```python
from build123d import *

# Parameters (mm, degrees)
SKETCH1_W           = 41
SKETCH1_H           = 19.4
BOSS_EXTRUDE1_DEPTH = 20.3
SKETCH2_W           = 54.7
SKETCH2_H           = 20.3
BOSS_EXTRUDE2_DEPTH = 2.6
SKETCH3_W           = 41
SKETCH3_H           = 20.3
BOSS_EXTRUDE3_DEPTH = 6.6
SKETCH4_R           = 2.2
CUT_EXTRUDE1_DEPTH  = 57.442116367
SKETCH5_R           = 5
BOSS_EXTRUDE4_DEPTH = 0.7
SKETCH6_R           = 2.97
BOSS_EXTRUDE5_DEPTH = 4.3


with BuildPart() as part:
    # Sketch1 → Boss-Extrude1 (new body)
    with BuildSketch(Plane.XY):
        with Locations((20.5, -9.7)):
            Rectangle(SKETCH1_W, SKETCH1_H)
    extrude(amount=BOSS_EXTRUDE1_DEPTH)

    # Sketch2 → Boss-Extrude2 (add)
    with BuildSketch(Plane(origin=(0, 0, 0), x_dir=(1, 0, 0), z_dir=(0, 1, 0))):
        with Locations((20.5, -10.15)):
            Rectangle(SKETCH2_W, SKETCH2_H)
    extrude(amount=BOSS_EXTRUDE2_DEPTH)

    # Sketch3 → Boss-Extrude3 (add)
    with BuildSketch(Plane(origin=(0, 2.6, 0), x_dir=(1, 0, 0), z_dir=(0, 1, 0))):
        with Locations((20.5, -10.15)):
            Rectangle(SKETCH3_W, SKETCH3_H)
    extrude(amount=BOSS_EXTRUDE3_DEPTH)

    # Sketch4 → Cut-Extrude1 (cut, through all)
    with BuildSketch(Plane(origin=(0, 2.6, 0), x_dir=(1, 0, 0), z_dir=(0, 1, 0))):
        with Locations(Location((-4.4, -15.15, 0), (0, 0, 270))):
            Circle(SKETCH4_R)
        with Locations(Location((-4.4, -5.15, 0), (0, 0, 270))):
            Circle(SKETCH4_R)
        with Locations(Location((45.4, -15.15, 0), (0, 0, 270))):
            Circle(SKETCH4_R)
        with Locations(Location((45.4, -5.15, 0), (0, 0, 270))):
            Circle(SKETCH4_R)
    extrude(amount=-CUT_EXTRUDE1_DEPTH, mode=Mode.SUBTRACT)

    # Sketch5 → Boss-Extrude4 (add)
    with BuildSketch(Plane(origin=(0, 9.2, 0), x_dir=(1, 0, 0), z_dir=(0, 1, 0))):
        with Locations(Location((32.1, -10.15, 0), (0, 0, 90))):
            Circle(SKETCH5_R)
    extrude(amount=BOSS_EXTRUDE4_DEPTH)

    # Sketch6 → Boss-Extrude5 (add)
    with BuildSketch(Plane(origin=(0, 9.9, 0), x_dir=(1, 0, 0), z_dir=(0, 1, 0))):
        with Locations(Location((32.1, -10.15, 0), (0, 0, 90))):
            Circle(SKETCH6_R)
    extrude(amount=BOSS_EXTRUDE5_DEPTH)


solid = part.part
```
Source: CAD feature listing. Evaluate the final solid. Frame: model axes, mm. A direction names the side the tool comes from. Round coordinates to 2 decimals unless told otherwise and drop trailing zeros. Loops run counter-clockwise (first coordinate to the right, second up) from the corner with the lowest first, then second, coordinate; pieces in that order, holes last.
1. Section query D-D on z = 14.5. Output: boundary loops of the cut face in (x, y).
2. Access query for faces 4 (the flat face through (0, 6, 10)), 5 (the flat face through (41, -10, 10)), 6 (the flat face through (41, 6, 10)). Directions: +Z, -Z, +X, -X, +Y, -Y. A direction counts if a zero-diameter tool reaches every point of the face in a straight line with its end or side. Return the directions, or none.
3. Ray query, L1, parallel to X at y = 1.4, z = 5.15; L2, parallel to Z at x = -4, y = 1; L3, parallel to X at y = -13, z = 4.75. Return the intervals inside material, ascending.
4. Section query B-B on z = 10.15. Output: boundary loops of the cut face in (x, y).
5. Contact query for flat-ended pins moving along their axis: pin 1 (6 mm diameter, centred on y = -9.5, z = 9, fed in from +X); pin 2 (10 mm diameter, centred on x = 11, z = 15, fed in from +Y); pin 3 (7.5 mm diameter, centred on y = 6.5, z = 12.5, fed in from -X); pin 4 (2.5 mm diameter, centred on x = -4.4, z = 5.15, fed in from -Y). Output: stop coordinate, or through.
6. Section query C-C on y = 12. Output: boundary loops of the cut face in (x, z).
7. Section query A-A on x = 45.4. Output: boundary loops of the cut face in (y, z), and give its area (3 significant figures).
8. Mould query, pull axis X, two halves, no side actions, for faces 1 (the flat face through (-3, 0, 10)), 2 (the flat face through (0, -10, 10)), 3 (the cylindrical face through (-4.303, 1.318, 12.952)). Classes: released by +X, released by -X, zero draft, split by the parting line, or undercut.
Answers below:
1. outline: (-6.85, 0) - (-6.5, 0) - (-6.5, 2.6) - (-6.85, 2.6) - close; (-2.3, 0) - (0, 0) - (0, -19.4) - (41, -19.4) - (41, 0) - (43.3, 0) - (43.3, 2.6) - (41, 2.6) - (41, 9.2) - (34.57, 9.2) - (34.57, 9.9) - (29.63, 9.9) - (29.63, 9.2) - (0, 9.2) - (0, 2.6) - (-2.3, 2.6) - close; (47.5, 0) - (47.85, 0) - (47.85, 2.6) - (47.5, 2.6) - close
2. face 4: +Z, -Z, -X, +Y
2. face 5: +Z, -Z, +X, -Y
2. face 6: +Z, -Z, +X, +Y
3. L1: x = -6.85 to -6.6, -2.2 to 43.2, 47.6 to 47.85
3. L2: z = 0 to 2.99, 7.31 to 12.99, 17.31 to 20.3
3. L3: x = 0 to 41
4. outline: (-6.85, 0) - (0, 0) - (0, -19.4) - (41, -19.4) - (41, 0) - (47.85, 0) - (47.85, 2.6) - (41, 2.6) - (41, 9.2) - (37.1, 9.2) - (37.1, 9.9) - (35.07, 9.9) - (35.07, 14.2) - (29.13, 14.2) - (29.13, 9.9) - (27.1, 9.9) - (27.1, 9.2) - (0, 9.2) - (0, 2.6) - (-6.85, 2.6) - close
5. pin 1: stops at x = 41
5. pin 2: stops at y = 9.2
5. pin 3: stops at x = 0
5. pin 4: passes through
6. outline: circle Ø5.94 at (32.1, 10.15)
7. outline: (0, 0) - (2.6, 0) - (2.6, 2.95) - (0, 2.95) - close; (0, 7.35) - (2.6, 7.35) - (2.6, 12.95) - (0, 12.95) - close; (0, 17.35) - (2.6, 17.35) - (2.6, 20.3) - (0, 20.3) - close
7. area: 29.9 mm2
8. face 1: zero draft
8. face 2: released by -X
8. face 3: undercut
